Geometry: final body of the model. Coordinates: model frame, mm. A direction names the side the tool comes from. Give positions to 0.01 mm unless a question says otherwise; leave off trailing zeros. Write each loop counter-clockwise with the first axis right and the second up, starting at its lowest first coordinate (ties: lowest second). Pieces come first, ordered by that corner, then holes.
Q1. Section C-C (z = 36). Return the cut outline in (x, y), plus the area to 3 significant figures.
Q2. Pin query (flat end, axial travel): pin 1 Ø2.5 at (y, z) = (0, 54) entering from +X; pin 2 Ø1.5 at (x, y) = (-7, 0) entering from +Z; pin 3 Ø3 at (x, y) = (8.5, -0.5) entering from +Z; pin 4 Ø1.8 at (y, z) = (-1, 54.5) entering from +X. Return the tip coordinate at first contact, or that it passes through.
Q3. Line query: line 1 (X direction, y = 0, z = 1.5); line 2 (Y direction, x = -7, z = 6.25); line 3 (Z direction, x = -11, y = 1.75). Output: solid intervals per line, ascending.
Q4. Mould query, pull axis Y, two halves, no side actions, for faces 5 (the flat face through (0, -3.5, 29)), 6 (the conical face through (7.22, 0.01, 8.12)), 7 (the cylindrical face through (-8.25, 0.05, 3.8)), 8 (the flat face through (0, 3.5, 29)). Classes: +Y half, -Y half, draft (parallel to the pull), parting line (faces both ways), or undercut.
Q5. Section B-B (x = 2). Return the cut outline in (y, z), plus the area to 3 significant figures.
Q6. Reachability of faces 1 (the flat face through (-5.5, 0.8, 55.4)), 2 (the flat face through (5.5, 0.8, 55.4)), 3 (the cylindrical face through (5.75, 0.05, 3.8)), 4 (the cylindrical face through (-11.93, -2.9, 25.35)) from +Z, -Z, +X, -X, +Y, -Y: full face, straight path, thin tool, end or side. Return the list, or none.
Q7. Section A-A (z = 54). Return the cut outline in (x, y).
from build123d import *

# Parameters (mm, degrees)
SKETCH1_W                 = 25
SKETCH1_H                 = 7
BOSS_EXTRUDE1_DEPTH       = 58
SKETCH2_W                 = 7
SKETCH2_H                 = 8
CUT_EXTRUDE1_DEPTH        = 60.74320045
M3X0_5_TAPPED_HOLE2_D     = 2.5
M3X0_5_TAPPED_HOLE2_DEPTH = 7.5
M3X0_5_TAPPED_HOLE2_TIP   = 0.751075774
CHAMFER1_SIZE             = 1
M2_5_CLEARANCE_HOLE1_D    = 2.9
FILLET1_R                 = 2
CHAMFER2_SIZE             = 1


with BuildPart() as part:
    # Sketch1 → Boss-Extrude1 (new body)
    with BuildSketch(Plane.XY):
        Rectangle(SKETCH1_W, SKETCH1_H)
    extrude(amount=BOSS_EXTRUDE1_DEPTH)

    # Sketch2 → Cut-Extrude1 (cut, through all)
    with BuildSketch(Plane(origin=(0, 3.5, 0), x_dir=(1, 0, 0), z_dir=(0, 1, 0))):
        with Locations((-9, -54)):
            Rectangle(SKETCH2_W, SKETCH2_H)
        with Locations((9, -54)):
            Rectangle(SKETCH2_W, SKETCH2_H)
    extrude(amount=-CUT_EXTRUDE1_DEPTH, mode=Mode.SUBTRACT)

    # M3x0.5 Tapped Hole2
    with Locations(Plane(origin=(0, 0, 0), x_dir=(-1, 0, 0), z_dir=(0, 0, -1))):
        with Locations((-7, 0), (7, 0)):
            Hole(M3X0_5_TAPPED_HOLE2_D / 2, depth=M3X0_5_TAPPED_HOLE2_DEPTH)
            with Locations((0, 0, -(M3X0_5_TAPPED_HOLE2_DEPTH + M3X0_5_TAPPED_HOLE2_TIP / 2))):  # 118° drill point
                Cone(0, M3X0_5_TAPPED_HOLE2_D / 2, M3X0_5_TAPPED_HOLE2_TIP, mode=Mode.SUBTRACT)

    # Chamfer1
    chamfer1_edges = [part.edges().sort_by_distance(p)[0] for p in [
        (-5.5, 0, 58),
        (5.5, 0, 58),
    ]]
    chamfer(chamfer1_edges, length=CHAMFER1_SIZE)

    # M2.5 Clearance Hole1 (through all)
    with Locations(Plane(origin=(-5.5, -6.575007997, -1.706532938), x_dir=(0, 0, 1), z_dir=(-1, 0, 0))):
        with Locations((55.706532938, 6.575007997)):
            Hole(M2_5_CLEARANCE_HOLE1_D / 2)

    # Fillet1
    fillet1_edges = [part.edges().sort_by_distance(p)[0] for p in [
        (-12.5, -3.5, 25),
        (-12.5, 3.5, 25),
        (12.5, -3.5, 25),
        (12.5, 3.5, 25),
    ]]
    fillet(fillet1_edges, radius=FILLET1_R)

    # Chamfer2
    chamfer2_edges = [part.edges().sort_by_distance(p)[0] for p in [
        (-5.5, 0, 50),
        (5.5, 0, 50),
    ]]
    chamfer(chamfer2_edges, length=CHAMFER2_SIZE)


solid = part.part
Computed:
1. outline: (-12.5, -1.5) arc R2 ccw to (-10.5, -3.5) - (10.5, -3.5) arc R2 ccw to (12.5, -1.5) - (12.5, 1.5) arc R2 ccw to (10.5, 3.5) - (-10.5, 3.5) arc R2 ccw to (-12.5, 1.5) - close
1. area: 172 mm2
2. pin 1: passes through
2. pin 2: stops at z = 50.25
2. pin 3: stops at z = 50
2. pin 4: stops at x = 5.5
3. line 1: x = -12.5 to -8.25, -5.75 to 5.75, 8.25 to 12.5
3. line 2: y = -3.5 to -1.25, 1.25 to 3.5
3. line 3: z = 0 to 50
4. face 5: -Y half
4. face 6: undercut
4. face 7: undercut
4. face 8: +Y half
5. outline: (-3.5, 0) - (3.5, 0) - (3.5, 58) - (-3.5, 58) - close; hole circle Ø2.9 at (0, 54)
5. area: 399 mm2
6. face 1: +Z, -X, +Y, -Y
6. face 2: +Z, +X, +Y, -Y
6. face 3: -Z
6. face 4: +Z, -Z, -X, -Y
7. outline: (-5.5, -3.5) - (5.5, -3.5) - (5.5, -1.45) - (-5.5, -1.45) - close; (-5.5, 1.45) - (5.5, 1.45) - (5.5, 3.5) - (-5.5, 3.5) - close
